Could you check a few things on this model? Use its own coordinates, in mm. Give positions to 0.01 mm unless a question says otherwise; leave off trailing zeros. Write each loop counter-clockwise with the first axis right and the second up, starting at its lowest first coordinate (ties: lowest second). Pieces come first, ordered by that corner, then holes. Notation, with made-up numbers: M -29.5,49.25 L -14.5,49.25 A14 cw -14.5,76.25 Z; hole C 4.25,-4.75 d11. An arc over 180 degrees is marked long. One line per item, written item: value.
```python
from build123d import *

# Parameters (mm, degrees)
SKETCH1_R           = 136.5
SKETCH1_R_2         = 2.25
BOSS_EXTRUDE1_DEPTH = 4.7


with BuildPart() as part:
    # Sketch1 → Boss-Extrude1 (new body)
    with BuildSketch(Plane(origin=(0, 0, 0), x_dir=(1, 0, 0), z_dir=(0, 1, 0))):
        Circle(SKETCH1_R)
        with Locations((-8, 77.66)):
            Circle(SKETCH1_R_2, mode=Mode.SUBTRACT)
        with Locations((8, 77.66)):
            Circle(SKETCH1_R_2, mode=Mode.SUBTRACT)
        with Locations((8, 61.66)):
            Circle(SKETCH1_R_2, mode=Mode.SUBTRACT)
        with Locations((-8, 61.66)):
            Circle(SKETCH1_R_2, mode=Mode.SUBTRACT)
        with Locations((-16, 22.54)):
            Circle(SKETCH1_R_2, mode=Mode.SUBTRACT)
        with Locations((16, 22.54)):
            Circle(SKETCH1_R_2, mode=Mode.SUBTRACT)
    extrude(amount=BOSS_EXTRUDE1_DEPTH)


solid = part.part
```
1) If we section it at B-B, the plane x = 39.5: Write out the boundary of the cut face in (y, z), then the cut area to 3 significant figures.
Outcome:
outline: M 0,-130.66 L 4.7,-130.66 L 4.7,130.66 L 0,130.66 Z
area: 1,230 mm^2
2) If we section it at C-C, the plane z = -33: Write out the boundary of the cut face in (x, y), then the cut area to 3 significant figures.
Outcome:
outline: M -132.45,0 L 132.45,0 L 132.45,4.7 L -132.45,4.7 Z
area: 1,250 mm^2
3) If we section it at A-A, the plane y = 1.3: Write out the boundary of the cut face in (x, z), then the cut area to 3 significant figures.
Outcome:
outline: C 0,0 d273; hole C -16,-22.54 d4.5; hole C -8,-77.66 d4.5; hole C -8,-61.66 d4.5; hole C 8,-77.66 d4.5; hole C 8,-61.66 d4.5; hole C 16,-22.54 d4.5
area: 58,400 mm^2
4) Please list where these lines run through material, in increasing order: L1, parallel to Z at x = -8, y = 1.1; L2, parallel to X at y = 3.6, z = -61.66; L3, parallel to X at y = 4, z = -63. Write a range as from..to.
Outcome:
L1: z = -136.27..-79.91, -75.41..-63.91, -59.41..136.27
L2: x = -121.78..-10.25, -5.75..5.75, 10.25..121.78
L3: x = -121.09..-9.81, -6.19..6.19, 9.81..121.09
